from build123d import *

# Parameters (mm, degrees)
BOSS_EXTRU_1_DEPTH       = 5
ESQUISSE2_W              = 80
ESQUISSE2_H              = 5
ENL_V_MAT_EXTRU_1_DEPTH  = 10
ESQUISSE3_R              = 2.5
ENL_V_MAT_EXTRU_6_DEPTH  = 2
ESQUISSE5_R              = 2.5
ENL_V_MAT_EXTRU_10_DEPTH = 2
ESQUISSE6_R              = 2.5
ENL_V_MAT_EXTRU_12_DEPTH = 6


with BuildPart() as part:
    # Esquisse1 → Boss.-Extru.1 (new body)
    with BuildSketch(Plane.XY):
        with BuildLine():
            Line((-79.721401665, 25), (-79.721401665, -10))
            Line((-79.721401665, -10), (-114.721401665, -10))
            ThreePointArc((-114.721401665, -10), (-114.995625295, -19.003076756), (-114.564392374, -28))
            Line((-114.564392374, -28), (-71.564392374, -28))
            Line((-71.564392374, -28), (-54.56, -76))
            Line((-54.56, -76), (54.56, -76))
            Line((54.56, -76), (71.564392374, -28))
            Line((71.564392374, -28), (114.564392374, -28))
            ThreePointArc((114.564392374, -28), (114.995625295, -19.003076756), (114.721401665, -10))
            Line((114.721401665, -10), (79.721401665, -10))
            Line((79.721401665, -10), (79.721401665, 25))
            Line((79.721401665, 25), (44.721401665, 25))
            Line((44.721401665, 25), (44.721401665, 40))
            Line((44.721401665, 40), (-44.721401665, 40))
            Line((-44.721401665, 40), (-44.721401665, 25))
            Line((-44.721401665, 25), (-79.721401665, 25))
        make_face()
        with BuildLine():
            ThreePointArc((-92.741576437, 50), (-115, -18), (-92.741576437, -86))
            Line((-92.741576437, -86), (-110.797111876, -86))
            ThreePointArc((-110.797111876, -86), (-130, -18), (-110.797111876, 50))
            Line((-110.797111876, 50), (-92.741576437, 50))
        make_face()
        with BuildLine():
            ThreePointArc((92.741576437, 50), (115, -18), (92.741576437, -86))
            Line((92.741576437, -86), (110.797111876, -86))
            ThreePointArc((110.797111876, -86), (130, -18), (110.797111876, 50))
            Line((110.797111876, 50), (92.741576437, 50))
        make_face()
    extrude(amount=BOSS_EXTRU_1_DEPTH)

    # Esquisse2 → Enlèv. mat.-Extru.1 (cut)
    with BuildSketch(Plane.XY.offset(5)):
        with Locations((0, 16)):
            Rectangle(ESQUISSE2_W, ESQUISSE2_H)
    extrude(amount=-ENL_V_MAT_EXTRU_1_DEPTH, mode=Mode.SUBTRACT)

    # Esquisse3 → Enlèv. mat.-Extru.6 (cut)
    with BuildSketch(Plane.XY.offset(5)):
        with Locations((-68, -19)):
            Circle(ESQUISSE3_R)
        with Locations((-78, -19)):
            Circle(ESQUISSE3_R)
    extrude(amount=-ENL_V_MAT_EXTRU_6_DEPTH, mode=Mode.SUBTRACT)

    # Esquisse5 → Enlèv. mat.-Extru.10 (cut)
    with BuildSketch(Plane.XY.offset(5)):
        with Locations((-29, -47)):
            Circle(ESQUISSE5_R)
        with Locations((-20.506096654, -67.506096654)):
            Circle(ESQUISSE5_R)
        with BuildLine():
            Line((-2.5, -76), (2.5, -76))
            ThreePointArc((2.5, -76), (0, -73.5), (-2.5, -76))
        make_face()
        with Locations((20.506096654, -67.506096654)):
            Circle(ESQUISSE5_R)
        with Locations((29, -47)):
            Circle(ESQUISSE5_R)
        with Locations((20.506096654, -26.493903346)):
            Circle(ESQUISSE5_R)
        with Locations((0, -18)):
            Circle(ESQUISSE5_R)
        with Locations((-20.506096654, -26.493903346)):
            Circle(ESQUISSE5_R)
    extrude(amount=-ENL_V_MAT_EXTRU_10_DEPTH, mode=Mode.SUBTRACT)

    # Esquisse6 → Enlèv. mat.-Extru.12 (cut, through all)
    with BuildSketch(Plane.XY.offset(5)):
        with Locations((-61.659877018, 0)):
            Circle(ESQUISSE6_R)
        with Locations((-44.659877018, 0)):
            Circle(ESQUISSE6_R)
        with Locations((-27.659877018, 0)):
            Circle(ESQUISSE6_R)
        with Locations((-10.659877018, 0)):
            Circle(ESQUISSE6_R)
        with Locations((6.340122982, 0)):
            Circle(ESQUISSE6_R)
        with Locations((23.340122982, 0)):
            Circle(ESQUISSE6_R)
        with Locations((40.340122982, 0)):
            Circle(ESQUISSE6_R)
        with Locations((57.340122982, 0)):
            Circle(ESQUISSE6_R)
        with Locations((-53.159877018, -15.034569708)):
            Circle(ESQUISSE6_R)
        with Locations((-36.159877018, -15.034569708)):
            Circle(ESQUISSE6_R)
        with Locations((-44.659877018, -33.372561191)):
            Circle(ESQUISSE6_R)
        with Locations((-44.659877018, -51.87866202)):
            Circle(ESQUISSE6_R)
        with Locations((44.659877018, -51.87866202)):
            Circle(ESQUISSE6_R)
        with Locations((44.659877018, -33.372561191)):
            Circle(ESQUISSE6_R)
        with Locations((36.159877018, -15.034569708)):
            Circle(ESQUISSE6_R)
        with Locations((53.159877018, -15.034569708)):
            Circle(ESQUISSE6_R)
    extrude(amount=-ENL_V_MAT_EXTRU_12_DEPTH, mode=Mode.SUBTRACT)


solid = part.part
Design review of the part built by this model. Coordinates are the model's own, in mm. A direction names the side the tool comes from. Round coordinates to 2 decimals unless told otherwise and drop trailing zeros. Order: outer loops, then holes, each group sorted by start corner. A loop starts at its lowest first (then second) coordinate and runs counter-clockwise, first axis right, second up.
1) Draft analysis for pull direction X (two halves, no side actions). For faces 5 (the flat face through (-2, -2, 5)), 6 (the cylindrical face through (-29.54, -49.44, 4.01)), state which applies: released by +X, released by -X, zero draft, split by the parting line, or undercut.
The answers:
face 5: zero draft
face 6: undercut
2) Consider section B-B (y = -47). State the section outline as (x, z) points.
The answers:
outline: (-126.72, 0) - (-111.28, 0) - (-111.28, 5) - (-126.72, 5) - close; (-64.83, 0) - (64.83, 0) - (64.83, 5) - (31.5, 5) - (31.5, 3) - (26.5, 3) - (26.5, 5) - (-26.5, 5) - (-26.5, 3) - (-31.5, 3) - (-31.5, 5) - (-64.83, 5) - close; (111.28, 0) - (126.72, 0) - (126.72, 5) - (111.28, 5) - close
3) Clearance check with flat-ended pins moving along their axes: pin 1 Ø4 at (x, y) = (-21.5, -67) entering from +Z; pin 2 Ø2.5 at (x, z) = (-10, 2) entering from -Y; pin 3 Ø0.8 at (x, y) = (-0.5, -74.5) entering from +Z; pin 4 Ø3 at (x, y) = (57.34, 0) entering from +Z. State where each tip first meets the part, or that it passes through.
The answers:
pin 1: stops at z = 5
pin 2: stops at y = -76
pin 3: stops at z = 3
pin 4: passes through
4) For L1, parallel to Y at x = 6, z = 3.4; L2, parallel to Y at x = 0, z = 3.7; L3, parallel to X at y = 32, z = 3.3, list the stretches that pass through material, from the lowest coordinate up.
The answers:
L1: y = -76 to -2.48, 2.48 to 13.5, 18.5 to 40
L2: y = -73.5 to -20.5, -15.5 to 13.5, 18.5 to 40
L3: x = -120 to -103.56, -44.72 to 44.72, 103.56 to 120
5) Consider section D-D (y = 28). State the section outline as (x, z) points, plus the area to 3 significant figures.
The answers:
outline: (-121.59, 0) - (-105.4, 0) - (-105.4, 5) - (-121.59, 5) - close; (-44.72, 0) - (44.72, 0) - (44.72, 5) - (-44.72, 5) - close; (105.4, 0) - (121.59, 0) - (121.59, 5) - (105.4, 5) - close
area: 609 mm2
6) Machinability: for faces 1 (the flat face through (102, 50, 2)), 2 (the flat face through (1, 40, 2)), 3 (the flat face through (97, -10, 2)), 4 (the flat face through (0, -18, 3)), which of the approach directions +Z, -Z, +X, -X, +Y, -Y give a long, thin tool a straight path to every point of the face, cutting with its end or side? Answer none if there is none.
The answers:
face 1: +Z, -Z, +X, -X, +Y
face 2: +Z, -Z, +Y
face 3: +Z, -Z
face 4: +Z
7) Consider section A-A (x = 29). State the section outline as (y, z) points.
The answers:
outline: (-76, 0) - (13.5, 0) - (13.5, 5) - (-44.5, 5) - (-44.5, 3) - (-49.5, 3) - (-49.5, 5) - (-76, 5) - close; (18.5, 0) - (40, 0) - (40, 5) - (18.5, 5) - close
8) Consider section C-C (x = 0). State the section outline as (y, z) points, plus the area to 3 significant figures.
The answers:
outline: (-76, 0) - (13.5, 0) - (13.5, 5) - (-15.5, 5) - (-15.5, 3) - (-20.5, 3) - (-20.5, 5) - (-73.5, 5) - (-73.5, 3) - (-76, 3) - close; (18.5, 0) - (40, 0) - (40, 5) - (18.5, 5) - close
area: 540 mm2
